Part model, mm, in its own coordinate system. A direction names the side the tool comes from. Round coordinates to 2 decimals unless told otherwise and drop trailing zeros. Loops run counter-clockwise (first coordinate to the right, second up) from the corner with the lowest first, then second, coordinate; pieces in that order, holes last. Notation, with made-up numbers: M 15,88.25 L 74,88.25 A14 cw 74,109.25 Z; hole C -27,60.25 d5. An arc over 180 degrees is marked long. Put each result on its own line as item: value. Start each with the question number.
1) Drop flat-ended pins along their axis: pin 1 Ø5 at (y, z) = (-60, 15) entering from +X; pin 2 Ø10 at (x, z) = (4, 12) entering from -Y; pin 3 Ø4 at (x, z) = (13, 21) entering from +Y. Give the stop position or say it passes through.
2) Slice it at C-C on y = 34. Give the cut face in (x, z), then the cut area to 3 significant figures.
3) Slice it at A-A on z = 3. Give the cut face in (x, y).
4) Slice it at B-B on x = -26.5. Give the cut face in (y, z), then the cut area to 3 significant figures.
5) Pull direction Y, two halves, no side cores. Call faces 6 (the flat face through (-12, 44.745, 26)), 7 (the flat face through (-12, 43.245, 25)), 8 (the flat face through (-48.953, -18, 26)): +Y half, -Y half, draft (parallel to the pull), parting line (faces both ways), or undercut.
6) Which spindle directions (+Z, -Z, +X, -X, +Y, -Y) get a long thin tool onto all of the face, cutting with end or side? Do faces 1 (the flat face through (-12, -16, 49)), 2 (the flat face through (26.047, -18, 26)), 3 (the flat face through (-12, -79.255, 26)), 4 (the flat face through (-12, -16, 50.5)), 5 (the flat face through (-50, -12, 0)). Say none if no direction does.
7) Probe line 1 along Y through (x, z) = (23, 40.5); line 2 along X through (y, z) = (39, 31.5); line 3 along Z through (x, y) = (11, -68.5). List the from-to ranges inside material, lowest first.
```python
from build123d import *

# Parameters (mm, degrees)
F0_W        = 75
F0_H        = 124
F1_DEPTH    = 50.5
F0_W_2      = 87
F0_H_2      = 136
F2_DEPTH    = 1.2
F3_T        = 1.5
F3_T3_DEPTH = 78
F3_T5_DEPTH = 127


# Not quite as in the source:
# - a shell that OpenCascade refuses in one call is made with other operations: the cavity is built on its own and cut out


with BuildPart() as f1:
    # F0 (on Top) → F1 (new body)
    with BuildSketch(Plane.XY):
        with Locations((-11.4526251853, -17.2550516479)):
            Rectangle(F0_W, F0_H)
    extrude(amount=F1_DEPTH)

    # F0 (on Top) → F2 (join)
    with BuildSketch(Plane.XY):
        with Locations((-11.4526251853, -17.2550516479)):
            Rectangle(F0_W_2, F0_H_2)
        with Locations((-11.4526251853, -17.2550516479)):
            Rectangle(F0_W, F0_H, mode=Mode.SUBTRACT)
    extrude(amount=F2_DEPTH)

    # F3: shell of thickness 1.5, made by hand


with BuildPart() as f3_core1:
    # F3_t2: copy of F1
    add(f1.part)

    # the walls: a layer under each face that stays
    f3_faces = [f3_core1.faces().sort_by_distance(p)[0] for p in [
        (-11.4526251853, 44.7449483521, 25.85),
        (-52.0526251853, -80.7217183146, 1.2),
        (-48.9526251853, -17.2550516479, 25.85),
        (-11.4526251853, -17.2550516479, 50.5),
        (26.0473748147, -17.2550516479, 25.85),
        (-11.4526251853, -85.2550516479, 0.6),
        (32.0473748147, -17.2550516479, 0.6),
        (-11.4526251853, 50.7449483521, 0.6),
        (-54.9526251853, -17.2550516479, 0.6),
        (-11.4526251853, -79.2550516479, 25.85),
    ]]
    thicken(f3_faces, amount=-F3_T, mode=Mode.SUBTRACT)

    # F3_s4 → F3_t3 (cut)
    with BuildSketch(Plane.YZ.offset(-50.4526251853)):
        Polygon((44.7599483521, 1.215), (43.2449483521, 1.2), (43.2449483521, -0.3), (44.7449483521, -0.3), align=None)
        Polygon((-79.2700516479, 1.215), (-79.2550516479, -0.3), (-77.7550516479, -0.3), (-77.7550516479, 1.2), align=None)
    extrude(amount=F3_T3_DEPTH, mode=Mode.SUBTRACT)

    # F3_s6 → F3_t5 (cut)
    with BuildSketch(Plane.XZ.offset(-46.2449483521)):
        Polygon((26.0623748147, 1.215), (26.0473748147, -0.3), (24.5473748147, -0.3), (24.5473748147, 1.2), align=None)
        Polygon((-48.9676251853, 1.215), (-48.9526251853, -0.3), (-47.4526251853, -0.3), (-47.4526251853, 1.2), align=None)
    extrude(amount=F3_T5_DEPTH, mode=Mode.SUBTRACT)


with BuildPart() as f1_1:
    add(f1.part)

    # what is left inside the walls is the cavity
    f3_cavity = [f3_core1.part.solids().sort_by_distance(p)[0] for p in [
        (-11.452625, -37.421718, 0.015),
    ]]
    add(f3_cavity, mode=Mode.SUBTRACT)


solid = f1_1.part
```
Recorded:
1. pin 1: stops at x = 26.05
1. pin 2: stops at y = -79.26
1. pin 3: stops at y = 44.74
2. outline: M -54.95,0 L -47.45,0 L -47.45,49 L 24.55,49 L 24.55,0 L 32.05,0 L 32.05,1.2 L 26.05,1.2 L 26.05,50.5 L -48.95,50.5 L -48.95,1.2 L -54.95,1.2 Z
2. area: 274 mm2
3. outline: M -48.95,-79.26 L 26.05,-79.26 L 26.05,44.74 L -48.95,44.74 Z; hole M -47.45,-77.76 L 24.55,-77.76 L 24.55,43.24 L -47.45,43.24 Z
4. outline: M -85.26,0 L -77.76,0 L -77.76,49 L 43.24,49 L 43.24,0 L 50.74,0 L 50.74,1.2 L 44.74,1.2 L 44.74,50.5 L -79.26,50.5 L -79.26,1.2 L -85.26,1.2 Z
4. area: 347 mm2
5. face 6: +Y half
5. face 7: undercut
5. face 8: draft
6. face 1: -Z
6. face 2: +Z, +X, +Y, -Y
6. face 3: +Z, +X, -X, -Y
6. face 4: +Z, +X, -X, +Y, -Y
6. face 5: -Z, +X, -X, +Y, -Y
7. line 1: y = -79.26 to -77.76, 43.24 to 44.74
7. line 2: x = -48.95 to -47.45, 24.55 to 26.05
7. line 3: z = 49 to 50.5
